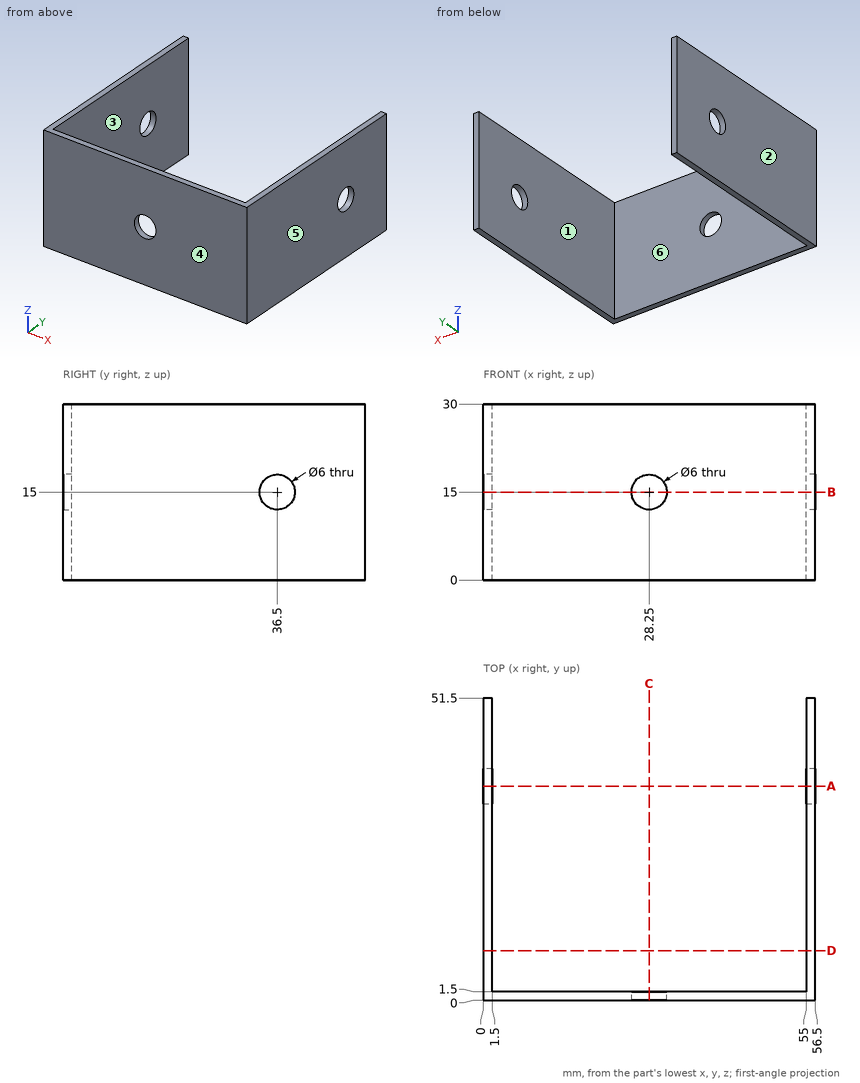
Source: three-view drawing plus pictorial views. Frame: mm from the lowest corner of the part. A direction names the side the tool comes from. Give positions to 0.01 mm unless a question says otherwise; leave off trailing zeros. Loops run counter-clockwise (first coordinate to the right, second up) from the corner with the lowest first, then second, coordinate; pieces in that order, holes last.
1) Section query D-D on y = 8.5. Return the cut outline in (x, z).
A:
outline: (0, 0) - (1.5, 0) - (1.5, 30) - (0, 30) - close; (55, 0) - (56.5, 0) - (56.5, 30) - (55, 30) - close
2) Section query A-A on y = 36.5. Return the cut outline in (x, z).
A:
outline: (0, 0) - (1.5, 0) - (1.5, 12) - (0, 12) - close; (0, 18) - (1.5, 18) - (1.5, 30) - (0, 30) - close; (55, 0) - (56.5, 0) - (56.5, 12) - (55, 12) - close; (55, 18) - (56.5, 18) - (56.5, 30) - (55, 30) - close
3) Reachability of the marked faces 5 and 6 from +Z, -Z, +X, -X, +Y, -Y: full face, straight path, thin tool, end or side. Return the list, or none.
A:
face 5: +Z, -Z, +X, +Y, -Y
face 6: +Z, -Z, +Y
4) Mould query, pull axis X, two halves, no side actions, for the marked faces 1, 2, 3 and 4. Classes: released by +X, released by -X, zero draft, split by the parting line, or undercut.
A:
face 1: undercut
face 2: released by -X
face 3: undercut
face 4: zero draft
5) Line query: L1, parallel to X at y = 19, z = 12.75; L2, parallel to Z at x = 0.85, y = 36.5; L3, parallel to X at y = 0.6, z = 15. Output: solid intervals per line, ascending.
A:
L1: x = 0 to 1.5, 55 to 56.5
L2: z = 0 to 12, 18 to 30
L3: x = 0 to 25.25, 31.25 to 56.5
6) Section query B-B on z = 15. Return the cut outline in (x, y), and give its area (3 significant figures).
A:
outline: (0, 0) - (25.25, 0) - (25.25, 1.5) - (1.5, 1.5) - (1.5, 33.5) - (0, 33.5) - close; (0, 39.5) - (1.5, 39.5) - (1.5, 51.5) - (0, 51.5) - close; (31.25, 0) - (56.5, 0) - (56.5, 33.5) - (55, 33.5) - (55, 1.5) - (31.25, 1.5) - close; (55, 39.5) - (56.5, 39.5) - (56.5, 51.5) - (55, 51.5) - close
area: 208 mm2
7) Contact query for a flat-ended pin moving along its axis: pin 1 (1 mm diameter, centred on x = 41.5, z = 4, fed in from +Y). Output: stop coordinate, or through.
A:
pin 1: stops at y = 1.5
8) Section query C-C on x = 28.25. Return the cut outline in (y, z), and give its area (3 significant figures).
A:
outline: (0, 0) - (1.5, 0) - (1.5, 12) - (0, 12) - close; (0, 18) - (1.5, 18) - (1.5, 30) - (0, 30) - close
area: 36.0 mm2
